Verification items for this drawing (mm, ordinates from the low corner). A direction names the side the tool comes from. Round coordinates to 2 decimals unless told otherwise and drop trailing zeros. Order: outer loops, then holes, each group sorted by start corner. A loop starts at its lowest first (then second) coordinate and runs counter-clockwise, first axis right, second up.
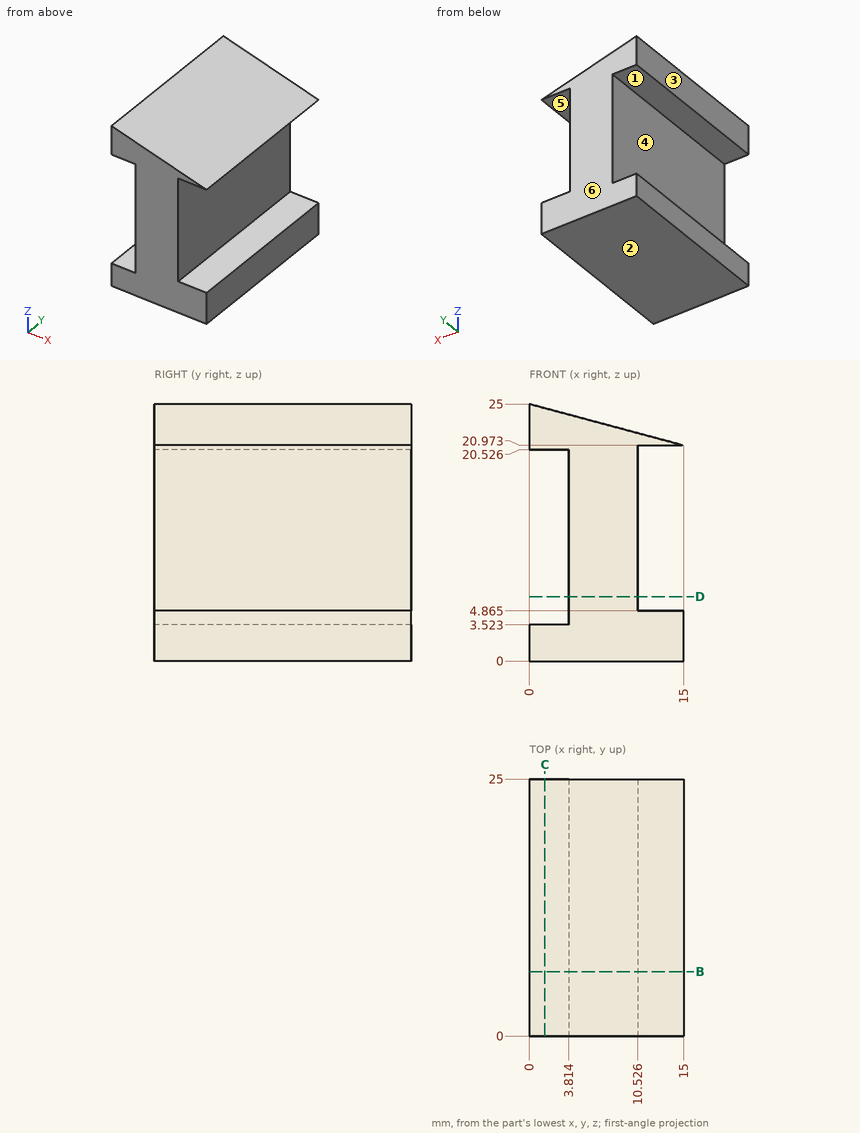
Item 1: Access from +Z, -Z, +X, -X, +Y, -Y to the whole of each face (thin tool, end or side, straight path). Record for the marked faces 4, 5 and 6.
Answer:
face 4: -X, +Y, -Y
face 5: +X, +Y, -Y
face 6: +Z, -Z, +X, -X, +Y
Item 2: Go/stop test with flat-tipped pins: P1, Ø3, axis at y = 9.5, z = 17.5, coming from the -X side; P2, Ø2, axis at x = 13, y = 6.5, coming from the +Z side; P3, Ø1, axis at x = 10.5, y = 10.5, coming from the +Z side (1 decimal); P4, Ø1.5, axis at x = 2, z = 17, coming from the +Y side. Record where each tip stops, or that it passes through.
Answer:
P1: stops at x = 3.81
P2: stops at z = 21.78
P3: stops at z = 22.3
P4: passes through
Item 3: Sectioned sample at D-D (z = 6.25). Record the cut outline in (x, y) (1 decimal).
Answer:
outline: (3.8, 0) - (10.5, 0) - (10.5, 25) - (3.8, 25) - close
Item 4: Scan lines: line 1 along X through (y, z) = (23.25, 18.75) (1 decimal); line 2 along Z through (x, y) = (12.25, 10) (1 decimal); line 3 along Z through (x, y) = (12.5, 21) (1 decimal). Record each from-to range of solid material in increasing order.
Answer:
line 1: x = 3.8 to 10.5
line 2: z = 0 to 4.9, 21 to 21.7
line 3: z = 0 to 4.9, 21 to 21.6
Item 5: Sectioned sample at C-C (x = 1.5). Record the cut outline in (y, z) (1 decimal), and give its area (3 significant figures).
Answer:
outline: (0, 0) - (25, 0) - (25, 3.5) - (0, 3.5) - close; (0, 20.5) - (25, 20.5) - (25, 24.6) - (0, 24.6) - close
area: 190 mm2
Item 6: Release check for a two-part mould opening along Z. For the marked faces 1, 2 and 3 record: released by +Z, released by -Z, zero draft, split by the parting line, or undercut.
Answer:
face 1: undercut
face 2: released by -Z
face 3: zero draft
Item 7: Sectioned sample at B-B (y = 6.25). Record the cut outline in (x, z) (1 decimal), and give its area (3 significant figures).
Answer:
outline: (0, 0) - (15, 0) - (15, 4.9) - (10.5, 4.9) - (10.5, 21) - (15, 21) - (0, 25) - (0, 20.5) - (3.8, 20.5) - (3.8, 3.5) - (0, 3.5) - close
area: 208 mm2
